```python
from build123d import *

# Parameters (mm, degrees)
F3_W          = 60
F3_H          = 91
F4_DEPTH      = 10
F5_W          = 56
F5_H          = 87
F5_W_2        = 24
F5_H_2        = 24
F6_DEPTH      = 8
F7_R          = 4
F8_DEPTH      = 10
F9_R          = 2
F10_DEPTH     = 10.001
F11_R         = 5
F12_R         = 5
F13_T1_DEPTH  = 77
F13_T3_DEPTH  = 14.5147186258
F13_T5_DEPTH  = 14.5147186258
F13_T8_ANGLE  = 90
F13_T10_ANGLE = 70.5287793655
F13_T12_ANGLE = 141.057558731
F13_T14_ANGLE = 90
F13_T16_ANGLE = 70.5287793655
F13_T18_ANGLE = 70.5287793655
F13_T20_ANGLE = 90
F13_T22_ANGLE = 141.057558731
F13_T24_ANGLE = 70.5287793655
F13_T26_ANGLE = 90
F13_T27_DEPTH = 81
F13_T29_DEPTH = 50
F13_T32_ANGLE = 90
F13_T34_ANGLE = 90
F13_T36_ANGLE = 90
F13_T38_ANGLE = 90
F14_R         = 8.5
F15_DEPTH     = 2.0010001
F16_DEPTH     = 10.0010001


# Not quite as in the source:
# - a fillet or chamfer that OpenCascade refuses, or shapes differently, is made with other operations: its cross-section is extruded or revolved along the edge and cut away or added


with BuildPart() as f4:
    # F3 (on Top) → F4 (new body)
    with BuildSketch(Plane.XY):
        Rectangle(F3_W, F3_H)
    extrude(amount=F4_DEPTH)

    # F5 (on face) → F6 (cut)
    with BuildSketch(Plane.XY.offset(10)):
        Rectangle(F5_W, F5_H)
        with Locations((0, 20.0242325664)):
            Rectangle(F5_W_2, F5_H_2, mode=Mode.SUBTRACT)
    extrude(amount=-F6_DEPTH, mode=Mode.SUBTRACT)

    # F7 (on face) → F8 (join)
    with BuildSketch(Plane(origin=(0, 0, 0), x_dir=(1, 0, 0), z_dir=(0, 0, -1))):
        with Locations((0, -41.5)):
            Circle(F7_R)
        with Locations((0, 41.5)):
            Circle(F7_R)
    extrude(amount=-F8_DEPTH)

    # F9 (on face) → F10 (cut, through all)
    with BuildSketch(Plane(origin=(0, 0, 0), x_dir=(1, 0, 0), z_dir=(0, 0, -1))):
        with Locations((0, -41.5)):
            Circle(F9_R)
        with Locations((0, 41.5)):
            Circle(F9_R)
    extrude(amount=-F10_DEPTH, mode=Mode.SUBTRACT)

    # F11
    f11_edges = [f4.edges().sort_by_distance(p)[0] for p in [
        (3.464102, 43.5, 6),
        (-3.464102, 43.5, 6),
        (-3.464102, -43.5, 6),
        (3.464102, -43.5, 6),
    ]]
    fillet(f11_edges, radius=F11_R)

    # F12
    f12_edges = [f4.edges().sort_by_distance(p)[0] for p in [
        (30, -45.5, 5),
        (-30, -45.5, 5),
        (30, 45.5, 5),
        (-30, 45.5, 5),
        (28, -43.5, 6),
        (-28, -43.5, 6),
        (-28, 43.5, 6),
        (28, 43.5, 6),
    ]]
    fillet(f12_edges, radius=F12_R)

    # F13: fillet of radius 3 on 24 edges, made by hand

    # F13_s2 → F13_t1 (join)
    with BuildSketch(Plane.XZ.offset(-38.5)):
        with BuildLine():
            ThreePointArc((-28, 5), (-27.1213203436, 2.8786796564), (-25, 2))
            Line((-25, 2), (-28, 2))
            Line((-28, 2), (-28, 5))
        make_face()
        with BuildLine():
            ThreePointArc((28, 5), (27.1213203436, 2.8786796564), (25, 2))
            Line((25, 2), (28, 2))
            Line((28, 2), (28, 5))
        make_face()
    extrude(amount=F13_T1_DEPTH)

    # F13_s4 → F13_t3 (join)
    with BuildSketch(Plane.YZ.offset(8.4852813742)):
        with BuildLine():
            ThreePointArc((-43.5, 5), (-42.6213203436, 2.8786796564), (-40.5, 2))
            Line((-40.5, 2), (-43.5, 2))
            Line((-43.5, 2), (-43.5, 5))
        make_face()
        with BuildLine():
            ThreePointArc((43.5, 5), (42.6213203436, 2.8786796564), (40.5, 2))
            Line((40.5, 2), (43.5, 2))
            Line((43.5, 2), (43.5, 5))
        make_face()
    extrude(amount=F13_T3_DEPTH)

    # F13_s6 → F13_t5 (join)
    with BuildSketch(Plane.YZ.offset(-23)):
        with BuildLine():
            ThreePointArc((-43.5, 5), (-42.6213203436, 2.8786796564), (-40.5, 2))
            Line((-40.5, 2), (-43.5, 2))
            Line((-43.5, 2), (-43.5, 5))
        make_face()
        with BuildLine():
            ThreePointArc((43.5, 5), (42.6213203436, 2.8786796564), (40.5, 2))
            Line((40.5, 2), (43.5, 2))
            Line((43.5, 2), (43.5, 5))
        make_face()
    extrude(amount=F13_T5_DEPTH)

    # F13_s7 → F13_t8 (revolve)
    with BuildSketch(Plane.YZ.offset(23)):
        with BuildLine():
            ThreePointArc((-43.5, 5), (-42.6213203436, 2.8786796564), (-40.5, 2))
            Line((-40.5, 2), (-43.5, 2))
            Line((-43.5, 2), (-43.5, 5))
        make_face()
    revolve(axis=Axis((23, -38.5, 2), (0, 0, 1)), revolution_arc=F13_T8_ANGLE)

    # F13_s9 → F13_t10 (revolve)
    with BuildSketch(Plane.YZ.offset(8.4852813742)):
        with BuildLine():
            ThreePointArc((-43.5, 5), (-42.6213203436, 2.8786796564), (-40.5, 2))
            Line((-40.5, 2), (-43.5, 2))
            Line((-43.5, 2), (-43.5, 5))
        make_face()
    revolve(axis=Axis((8.4852813742, -38.5, 2), (0, 0, -1)), revolution_arc=F13_T10_ANGLE)

    # F13_s11 → F13_t12 (revolve)
    with BuildSketch(Plane(origin=(-13.0421917419, -36.8888888889, 0), x_dir=(0, 0, 1), z_dir=(-0.3333333333, -0.9428090416, 0))):
        with BuildLine():
            ThreePointArc((5, -9.8333333333), (2.8786796564, -8.9546536769), (2, -6.8333333333))
            Line((2, -6.8333333333), (2, -9.8333333333))
            Line((2, -9.8333333333), (5, -9.8333333333))
        make_face()
    revolve(axis=Axis((0, -41.5, 2), (0, 0, -1)), revolution_arc=F13_T12_ANGLE)

    # F13_s13 → F13_t14 (revolve)
    with BuildSketch(Plane.XZ.offset(-38.5)):
        with BuildLine():
            ThreePointArc((28, 5), (27.1213203436, 2.8786796564), (25, 2))
            Line((25, 2), (28, 2))
            Line((28, 2), (28, 5))
        make_face()
    revolve(axis=Axis((23, 38.5, 2), (0, 0, 1)), revolution_arc=F13_T14_ANGLE)

    # F13_s15 → F13_t16 (revolve)
    with BuildSketch(Plane(origin=(-13.0421917419, -36.8888888889, 0), x_dir=(0, 0, 1), z_dir=(0.3333333333, 0.9428090416, 0))):
        with BuildLine():
            ThreePointArc((5, 9.8333333333), (2.8786796564, 8.9546536769), (2, 6.8333333333))
            Line((2, 6.8333333333), (2, 9.8333333333))
            Line((2, 9.8333333333), (5, 9.8333333333))
        make_face()
    revolve(axis=Axis((-8.4852813742, -38.5, 2), (0, 0, -1)), revolution_arc=F13_T16_ANGLE)

    # F13_s17 → F13_t18 (revolve)
    with BuildSketch(Plane.YZ.offset(8.4852813742)):
        with BuildLine():
            ThreePointArc((43.5, 5), (42.6213203436, 2.8786796564), (40.5, 2))
            Line((40.5, 2), (43.5, 2))
            Line((43.5, 2), (43.5, 5))
        make_face()
    revolve(axis=Axis((8.4852813742, 38.5, 2), (0, 0, 1)), revolution_arc=F13_T18_ANGLE)

    # F13_s19 → F13_t20 (revolve)
    with BuildSketch(Plane.YZ.offset(-23)):
        with BuildLine():
            ThreePointArc((-43.5, 5), (-42.6213203436, 2.8786796564), (-40.5, 2))
            Line((-40.5, 2), (-43.5, 2))
            Line((-43.5, 2), (-43.5, 5))
        make_face()
    revolve(axis=Axis((-23, -38.5, 2), (0, 0, -1)), revolution_arc=F13_T20_ANGLE)

    # F13_s21 → F13_t22 (revolve)
    with BuildSketch(Plane(origin=(13.0421917419, 36.8888888889, 0), x_dir=(0, 0, 1), z_dir=(0.3333333333, 0.9428090416, 0))):
        with BuildLine():
            ThreePointArc((5, -9.8333333333), (2.8786796564, -8.9546536769), (2, -6.8333333333))
            Line((2, -6.8333333333), (2, -9.8333333333))
            Line((2, -9.8333333333), (5, -9.8333333333))
        make_face()
    revolve(axis=Axis((0, 41.5, 2), (0, 0, -1)), revolution_arc=F13_T22_ANGLE)

    # F13_s23 → F13_t24 (revolve)
    with BuildSketch(Plane(origin=(-13.0421917419, 36.8888888889, 0), x_dir=(0, 0, 1), z_dir=(0.3333333333, -0.9428090416, 0))):
        with BuildLine():
            ThreePointArc((5, -9.8333333333), (2.8786796564, -8.9546536769), (2, -6.8333333333))
            Line((2, -6.8333333333), (2, -9.8333333333))
            Line((2, -9.8333333333), (5, -9.8333333333))
        make_face()
    revolve(axis=Axis((-8.4852813742, 38.5, 2), (0, 0, 1)), revolution_arc=F13_T24_ANGLE)

    # F13_s25 → F13_t26 (revolve)
    with BuildSketch(Plane.XZ.offset(-38.5)):
        with BuildLine():
            ThreePointArc((-28, 5), (-27.1213203436, 2.8786796564), (-25, 2))
            Line((-25, 2), (-28, 2))
            Line((-28, 2), (-28, 5))
        make_face()
    revolve(axis=Axis((-23, 38.5, 2), (0, 0, -1)), revolution_arc=F13_T26_ANGLE)

    # F13_s28 → F13_t27 (cut)
    with BuildSketch(Plane.XZ.offset(-40.5)):
        with BuildLine():
            ThreePointArc((30, 3), (29.1213203436, 0.8786796564), (27, 0))
            Line((27, 0), (30, 0))
            Line((30, 0), (30, 3))
        make_face()
        with BuildLine():
            ThreePointArc((-30, 3), (-29.1213203436, 0.8786796564), (-27, 0))
            Line((-27, 0), (-30, 0))
            Line((-30, 0), (-30, 3))
        make_face()
    extrude(amount=F13_T27_DEPTH, mode=Mode.SUBTRACT)

    # F13_s30 → F13_t29 (cut)
    with BuildSketch(Plane.YZ.offset(-25)):
        with BuildLine():
            ThreePointArc((-45.5, 3), (-44.6213203436, 0.8786796564), (-42.5, 0))
            Line((-42.5, 0), (-45.5, 0))
            Line((-45.5, 0), (-45.5, 3))
        make_face()
        with BuildLine():
            ThreePointArc((45.5, 3), (44.6213203436, 0.8786796564), (42.5, 0))
            Line((42.5, 0), (45.5, 0))
            Line((45.5, 0), (45.5, 3))
        make_face()
    extrude(amount=F13_T29_DEPTH, mode=Mode.SUBTRACT)

    # F13_s31 → F13_t32 (revolve, cut)
    with BuildSketch(Plane.YZ.offset(25)):
        with BuildLine():
            ThreePointArc((-45.5, 3), (-44.6213203436, 0.8786796564), (-42.5, 0))
            Line((-42.5, 0), (-45.5, 0))
            Line((-45.5, 0), (-45.5, 3))
        make_face()
    revolve(axis=Axis((25, -40.5, 0), (0, 0, 1)), revolution_arc=F13_T32_ANGLE, mode=Mode.SUBTRACT)

    # F13_s33 → F13_t34 (revolve, cut)
    with BuildSketch(Plane.YZ.offset(-25)):
        with BuildLine():
            ThreePointArc((-45.5, 3), (-44.6213203436, 0.8786796564), (-42.5, 0))
            Line((-42.5, 0), (-45.5, 0))
            Line((-45.5, 0), (-45.5, 3))
        make_face()
    revolve(axis=Axis((-25, -40.5, 0), (0, 0, -1)), revolution_arc=F13_T34_ANGLE, mode=Mode.SUBTRACT)

    # F13_s35 → F13_t36 (revolve, cut)
    with BuildSketch(Plane.XZ.offset(-40.5)):
        with BuildLine():
            ThreePointArc((30, 3), (29.1213203436, 0.8786796564), (27, 0))
            Line((27, 0), (30, 0))
            Line((30, 0), (30, 3))
        make_face()
    revolve(axis=Axis((25, 40.5, 0), (0, 0, 1)), revolution_arc=F13_T36_ANGLE, mode=Mode.SUBTRACT)

    # F13_s37 → F13_t38 (revolve, cut)
    with BuildSketch(Plane.XZ.offset(-40.5)):
        with BuildLine():
            ThreePointArc((-30, 3), (-29.1213203436, 0.8786796564), (-27, 0))
            Line((-27, 0), (-30, 0))
            Line((-30, 0), (-30, 3))
        make_face()
    revolve(axis=Axis((-25, 40.5, 0), (0, 0, -1)), revolution_arc=F13_T38_ANGLE, mode=Mode.SUBTRACT)

    # F14 (on face) → F15 (cut, through all)
    with BuildSketch(Plane.XY.offset(2)):
        with Locations((11.5, -24.7238390148)):
            Circle(F14_R)
        with Locations((-11.5, -24.7238390148)):
            Circle(F14_R)
    extrude(amount=-F15_DEPTH, mode=Mode.SUBTRACT)

    # F16 (cut, through all): a face of the model
    f16_faces = [f4.faces().sort_by_distance(p)[0] for p in [
        (0, 20.0242325664, 10),
    ]]
    extrude(f16_faces, amount=-F16_DEPTH, mode=Mode.SUBTRACT)


solid = f4.part
```
Build history of the part. All positions in model axes, mm. A direction names the side the tool comes from. Round coordinates to 2 decimals unless told otherwise and drop trailing zeros. Loops run counter-clockwise (first coordinate to the right, second up) from the corner with the lowest first, then second, coordinate; pieces in that order, holes last. Notation, with made-up numbers: M -5,45 L 52,45 A27 cw 52,65 Z; hole C 13,4 d2. An arc over 180 degrees is marked long. Answer as CSV lines item,"result".
1. Wall check: probe 1 along Y at (x, z) = (0, 7.75); probe 2 along X at (y, z) = (-29, 6.75); probe 3 along X at (y, z) = (-41.5, 8.25). Give the ranges that are in metal, low to high. Write a range as [from, to].
Resolved:
probe 1,"y = [-45.5, -43.5], [-39.5, -37.5], [37.5, 39.5], [43.5, 45.5]"
probe 2,"x = [-30, -28], [28, 30]"
probe 3,"x = [-29.9, -27], [-4.49, -2], [2, 4.49], [27, 29.9]"
2. Cut at C-C on z = 7. Write the cut outline in (x, y).
Resolved:
outline,"M -30,-40.5 A5 ccw -25,-45.5 L 25,-45.5 A5 ccw 30,-40.5 L 30,40.5 A5 ccw 25,45.5 L -25,45.5 A5 ccw -30,40.5 Z; hole M -28,-38.5 A5 ccw -23,-43.5 L -8.49,-43.5 A5 ccw -3.77,-40.17 A4 cw 3.77,-40.17 A5 ccw 8.49,-43.5 L 23,-43.5 A5 ccw 28,-38.5 L 28,38.5 A5 ccw 23,43.5 L 8.49,43.5 A5 ccw 3.77,40.17 A4 cw -3.77,40.17 A5 ccw -8.49,43.5 L -23,43.5 A5 ccw -28,38.5 Z; hole C 0,-41.5 d4; hole C 0,41.5 d4"
3. 3-axis set-ups, long thin cutter, end or side, ignore diameter. For faces 1 (the flat face through (0, 32.024, 1)), 2 (the flat face through (0, 1, 0)), 3 (the cylindrical face through (-26.5, 42.07, 7.46)): which of +Z, -Z, +X, -X, +Y, -Y reach the whole face in a straight line?
Resolved:
face 1,"+Z, -Z"
face 2,"-Z, +X, -X, +Y, -Y"
face 3,"+Z"
4. Cut at B-B on x = 16. Write the cut outline in (y, z), then the cut area to 3 significant figures.
Resolved:
outline,"M -45.5,3 A3 ccw -42.5,0 L -31.93,0 L -31.93,2 L -40.5,2 A3 cw -43.5,5 L -43.5,10 L -45.5,10 Z; M -17.51,0 L 42.5,0 A3 ccw 45.5,3 L 45.5,10 L 43.5,10 L 43.5,5 A3 cw 40.5,2 L -17.51,2 Z"
area,"185 mm²"
5. Cut at D-D on y = -12.5. Write the cut outline in (x, z), then the cut area to 3 significant figures.
Resolved:
outline,"M -30,3 A3 ccw -27,0 L 27,0 A3 ccw 30,3 L 30,10 L 28,10 L 28,5 A3 cw 25,2 L -25,2 A3 cw -28,5 L -28,10 L -30,10 Z"
area,"152 mm²"
6. Cut at A-A on y = 24. Write the cut outline in (x, z), then the cut area to 3 significant figures.
Resolved:
outline,"M -30,3 A3 ccw -27,0 L -12,0 L -12,2 L -25,2 A3 cw -28,5 L -28,10 L -30,10 Z; M 12,0 L 27,0 A3 ccw 30,3 L 30,10 L 28,10 L 28,5 A3 cw 25,2 L 12,2 Z"
area,"104 mm²"
7. Two-plate mould, pull along X, no slides. Class faces 4 (the cylindrical face through (27.14, 0.54, 2.9)), 5 (the cylindrical face through (-28.57, -44, 6.55)), 6 (the flat face through (-29, 0, 10)), 7 (the cylindrical face through (28.5, 44.07, 6.55)): released by +X, released by -X, zero draft, split by the parting line, or undercut.
Resolved:
face 4,"undercut"
face 5,"released by -X"
face 6,"zero draft"
face 7,"released by +X"
8. Flat gauge pins, fed straight in: P1, Ø3, axis at x = -23.5, y = -30, coming from the +Z side; P2, Ø1.6, axis at x = 2, z = 1.5, coming from the -Y side; P3, Ø1.6, axis at x = -1, z = 1, coming from the +Y side; P4, Ø15.5, axis at x = 11.5, y = -24.72, coming from the +Z side. Where does each tip first touch, or does it go through?
Resolved:
P1,"stops at z = 2"
P2,"stops at y = -45.42"
P3,"stops at y = 45.25"
P4,"passes through"
